from build123d import *

# Parameters (mm, degrees)
IZIM1_W                      = 50.7
IZIM1_H                      = 48.2
Y_KSEKLIK_EKSTR_ZYON1_DEPTH  = 26.7
IZIM2_R                      = 8.7
Y_KSEKLIK_EKSTR_ZYON2_DEPTH  = 0.5
Y_KSEKLIK_EKSTR_ZYON3_DEPTH  = 11.9
IZIM4_R                      = 16.5
Y_KSEKLIK_EKSTR_ZYON4_DEPTH  = 0.9
IZIM5_R                      = 18
Y_KSEKLIK_EKSTR_ZYON5_DEPTH  = 0.9
Y_KSEKLIK_EKSTR_ZYON6_DEPTH  = 36
Y_KSEKLIK_EKSTR_ZYON7_DEPTH  = 17
Y_KSEKLIK_EKSTR_ZYON8_START  = 17
Y_KSEKLIK_EKSTR_ZYON8_DEPTH  = 17
IZIM9_W                      = 14.75
IZIM9_H                      = 70
KES_EKSTR_ZYON1_DEPTH        = 30.160746911
IZIM10_W                     = 14.75
IZIM10_H                     = 70
KES_EKSTR_ZYON2_DEPTH        = 30.160746911
IZIM11_W                     = 50.7
IZIM11_H                     = 48.2
Y_KSEKLIK_EKSTR_ZYON9_DEPTH  = 9.3
Y_KSEKLIK_EKSTR_ZYON10_START = 20
Y_KSEKLIK_EKSTR_ZYON10_DEPTH = 20
IZIM13_W                     = 9.75
IZIM13_H                     = 10.2
Y_KSEKLIK_EKSTR_ZYON11_DEPTH = 26.5
Y_KSEKLIK_EKSTR_ZYON12_DEPTH = 42.2
Y_KSEKLIK_EKSTR_ZYON13_START = -42.2
Y_KSEKLIK_EKSTR_ZYON13_DEPTH = 42.2
IZIM16_W                     = 29
IZIM16_H                     = 34.79
Y_KSEKLIK_EKSTR_ZYON14_DEPTH = 9.9
Y_KSEKLIK_EKSTR_ZYON15_DEPTH = 8.5
Y_KSEKLIK_EKSTR_ZYON16_DEPTH = 8.5
IZIM19_W                     = 6.3
IZIM19_H                     = 0.8
Y_KSEKLIK_EKSTR_ZYON17_DEPTH = 12
DRAFT1_ANGLE                 = 50
IZIM20_W                     = 5
IZIM20_H                     = 7.5
IZIM21_W                     = 5
IZIM21_H                     = 7.5
IZIM22_W                     = 5
IZIM22_H                     = 7.5
IZIM23_W                     = 5
IZIM23_H                     = 7.5
IZIM24_W                     = 5.2
IZIM24_H                     = 2.6
M20_BO_LUKLU_DELIK1_D        = 24
M20_BO_LUKLU_DELIK1_DEPTH    = 33.25
M27_BO_LUKLU_DELIK2_D        = 30.291
M27_BO_LUKLU_DELIK2_DEPTH    = 33.249
FEDER1_START                 = -30
FEDER1_DEPTH                 = 9.75
PAH1_SIZE                    = 1.479
RADYUS1_R                    = 0.8
RADYUS2_R                    = 2
RADYUS3_R                    = 5
RADYUS4_R                    = 5.1
RADYUS5_R                    = 7
RADYUS6_R                    = 8.16
L_EK1_SCALE                  = 0.31


# Read off the part's stored shape, not the designer's step: Feder1
with BuildPart() as part:
    # Çizim1 → Yükseklik-Ekstrüzyon1 (new body)
    with BuildSketch(Plane(origin=(18, 0, 0), x_dir=(0, 0, -1), z_dir=(1, 0, 0))):
        with Locations((-0.35, 68.8)):
            Rectangle(IZIM1_W, IZIM1_H)
    extrude(amount=-Y_KSEKLIK_EKSTR_ZYON1_DEPTH)

    # Çizim2 → Yükseklik-Ekstrüzyon2 (add)
    with BuildSketch(Plane.XZ.offset(-44.7)):
        with Locations(Location((0, 0, 0), (0, 0, 180))):
            Circle(IZIM2_R)
    extrude(amount=Y_KSEKLIK_EKSTR_ZYON2_DEPTH)

    # Çizim3 → Yükseklik-Ekstrüzyon3 (add)
    with BuildSketch(Plane(origin=(0, 44.2, 0), x_dir=(1, 0, 0), z_dir=(0, 1, 0))):
        Polygon((-18, 10.392304845), (-18, -10.392304845), (0, -20.784609691), (18, -10.392304845), (18, 10.392304845), (0, 20.784609691), align=None)
    extrude(amount=-Y_KSEKLIK_EKSTR_ZYON3_DEPTH)

    # Çizim4 → Yükseklik-Ekstrüzyon4 (add)
    with BuildSketch(Plane.XZ.offset(-32.3)):
        with Locations(Location((0, 0, 0), (0, 0, 270))):
            Circle(IZIM4_R)
    extrude(amount=Y_KSEKLIK_EKSTR_ZYON4_DEPTH)

    # Çizim5 → Yükseklik-Ekstrüzyon5 (add)
    with BuildSketch(Plane(origin=(0, 31.4, 0), x_dir=(1, 0, 0), z_dir=(0, 1, 0))):
        with Locations(Location((0, 0, 0), (0, 0, 90))):
            Circle(IZIM5_R)
    extrude(amount=-Y_KSEKLIK_EKSTR_ZYON5_DEPTH)

    # Çizim6 → Yükseklik-Ekstrüzyon6 (add)
    with BuildSketch(Plane.XY.offset(18)):
        with BuildLine():
            Line((-13.564659966, -21), (13.564659966, -21))
            ThreePointArc((13.564659966, -21), (17.201870235, -18.14099392), (20.25, -14.660746911))
            Line((20.25, -14.660746911), (35, -14.660746911))
            Line((35, -14.660746911), (35, 30.5))
            Line((35, 30.5), (0, 30.5))
            Line((0, 30.5), (-35, 30.5))
            Line((-35, 30.5), (-35, -14.660746911))
            Line((-35, -14.660746911), (-20.25, -14.660746911))
            ThreePointArc((-20.25, -14.660746911), (-17.201870235, -18.14099392), (-13.564659966, -21))
        make_face()
    extrude(amount=-Y_KSEKLIK_EKSTR_ZYON6_DEPTH)

    # Çizim7 → Yükseklik-Ekstrüzyon7 (add)
    with BuildSketch(Plane(origin=(0, 0, -18), x_dir=(-1, 0, 0), z_dir=(0, 0, -1))):
        with BuildLine():
            Line((13.564659966, -21), (-13.564659966, -21))
            ThreePointArc((-13.564659966, -21), (-17.201870235, -18.14099392), (-20.25, -14.660746911))
            Line((-20.25, -14.660746911), (-35, -14.660746911))
            Line((-35, -14.660746911), (-35, 30.5))
            Line((-35, 30.5), (35, 30.5))
            Line((35, 30.5), (35, -14.660746911))
            Line((35, -14.660746911), (20.25, -14.660746911))
            ThreePointArc((20.25, -14.660746911), (17.201870235, -18.14099392), (13.564659966, -21))
        make_face()
    extrude(amount=Y_KSEKLIK_EKSTR_ZYON7_DEPTH)

    # Çizim8 → Yükseklik-Ekstrüzyon8 (add)
    with BuildSketch(Plane.XY.offset(18).offset(Y_KSEKLIK_EKSTR_ZYON8_START)):
        with BuildLine():
            Line((13.564659966, -21), (-13.564659966, -21))
            ThreePointArc((-13.564659966, -21), (-17.201870235, -18.14099392), (-20.25, -14.660746911))
            Line((-20.25, -14.660746911), (-35, -14.660746911))
            Line((-35, -14.660746911), (-35, 30.5))
            Line((-35, 30.5), (35, 30.5))
            Line((35, 30.5), (35, -14.660746911))
            Line((35, -14.660746911), (20.25, -14.660746911))
            ThreePointArc((20.25, -14.660746911), (17.201870235, -18.14099392), (13.564659966, -21))
        make_face()
    extrude(amount=-Y_KSEKLIK_EKSTR_ZYON8_DEPTH)

    # Çizim9 → Kes-Ekstrüzyon1 (cut)
    with BuildSketch(Plane.XZ.offset(14.660746911)):
        with Locations((27.625, 0)):
            Rectangle(IZIM9_W, IZIM9_H)
    extrude(amount=-KES_EKSTR_ZYON1_DEPTH, mode=Mode.SUBTRACT)

    # Çizim10 → Kes-Ekstrüzyon2 (cut)
    with BuildSketch(Plane.XZ.offset(14.660746911)):
        with Locations((-27.625, 0)):
            Rectangle(IZIM10_W, IZIM10_H)
    extrude(amount=-KES_EKSTR_ZYON2_DEPTH, mode=Mode.SUBTRACT)

    # Çizim11 → Yükseklik-Ekstrüzyon9 (add)
    with BuildSketch(Plane.ZY.offset(8.7)):
        with Locations((0.35, 68.8)):
            Rectangle(IZIM11_W, IZIM11_H)
    extrude(amount=Y_KSEKLIK_EKSTR_ZYON9_DEPTH)

    # Çizim12 → Yükseklik-Ekstrüzyon10 (add)
    with BuildSketch(Plane.XY.offset(35).offset(Y_KSEKLIK_EKSTR_ZYON10_START)):
        with BuildLine():
            Line((-20.25, -14.660746911), (-20.25, 17.715834237))
            ThreePointArc((-20.25, 17.715834237), (0, 22), (20.25, 17.715834237))
            Line((20.25, 17.715834237), (20.25, -14.660746911))
            ThreePointArc((20.25, -14.660746911), (17.201870235, -18.14099392), (13.564659966, -21))
            Line((13.564659966, -21), (-13.564659966, -21))
            ThreePointArc((-13.564659966, -21), (-17.201870235, -18.14099392), (-20.25, -14.660746911))
        make_face()
    extrude(amount=-Y_KSEKLIK_EKSTR_ZYON10_DEPTH)

    # Çizim13 → Yükseklik-Ekstrüzyon11 (add)
    with BuildSketch(Plane.XZ.offset(-15.5)):
        with Locations((25.125, 15.1)):
            Rectangle(IZIM13_W, IZIM13_H)
    extrude(amount=Y_KSEKLIK_EKSTR_ZYON11_DEPTH)

    # Çizim14 → Yükseklik-Ekstrüzyon12 (add)
    with BuildSketch(Plane(origin=(0, 89.9, 0), x_dir=(1, 0, 0), z_dir=(0, 1, 0))):
        with BuildLine():
            Line((-18, -8.717797887), (-18, 8.717797887))
            ThreePointArc((-18, 8.717797887), (-20, 0), (-18, -8.717797887))
        make_face()
    extrude(amount=-Y_KSEKLIK_EKSTR_ZYON12_DEPTH)

    # Çizim15 → Yükseklik-Ekstrüzyon13 (add)
    with BuildSketch(Plane.XZ.offset(-47.7).offset(Y_KSEKLIK_EKSTR_ZYON13_START)):
        with BuildLine():
            Line((18, 8.717797887), (18, -8.717797887))
            ThreePointArc((18, -8.717797887), (20, 0), (18, 8.717797887))
        make_face()
    extrude(amount=Y_KSEKLIK_EKSTR_ZYON13_DEPTH)

    # Çizim16 → Yükseklik-Ekstrüzyon14 (add)
    with BuildSketch(Plane.XY.offset(25.7)):
        with Locations((0, 75.495)):
            Rectangle(IZIM16_W, IZIM16_H)
    extrude(amount=Y_KSEKLIK_EKSTR_ZYON14_DEPTH)

    # Çizim17 → Yükseklik-Ekstrüzyon15 (add)
    with BuildSketch(Plane.XY.offset(35.6)):
        Polygon((-9.4, 81.4), (-7.6, 81.4), (-7.6, 80.6), (-8.6, 80.6), (-8.6, 77.4), (-7.6, 77.4), (-7.6, 76.6), (-9.4, 76.6), align=None)
    extrude(amount=Y_KSEKLIK_EKSTR_ZYON15_DEPTH)

    # Çizim18 → Yükseklik-Ekstrüzyon16 (add)
    with BuildSketch(Plane.XY.offset(35.6)):
        Polygon((7.6, 77.4), (8.6, 77.4), (8.6, 80.6), (7.6, 80.6), (7.6, 81.4), (9.4, 81.4), (9.4, 76.6), (7.6, 76.6), align=None)
    extrude(amount=Y_KSEKLIK_EKSTR_ZYON16_DEPTH)

    # Çizim19 → Yükseklik-Ekstrüzyon17 (add)
    with BuildSketch(Plane.XY.offset(35.6)):
        with Locations((0, 70)):
            Rectangle(IZIM19_W, IZIM19_H)
    extrude(amount=Y_KSEKLIK_EKSTR_ZYON17_DEPTH)

    # Draft1
    draft1_faces = [part.faces().sort_by_distance(p)[0] for p in [
        (25.125, 2.25, 10),
    ]]
    draft(draft1_faces, Plane(origin=(0, -11, 0), x_dir=(0, 0, -1), z_dir=(0, -1, 0)), DRAFT1_ANGLE)

    # Çizim20 → Döndür1 (revolve)
    with BuildSketch(Plane.XY.offset(26.25), mode=Mode.PRIVATE) as d_nd_r1_sk:
        with Locations((-23.75, 34.25)):
            Rectangle(IZIM20_W, IZIM20_H)
    revolve(d_nd_r1_sk.sketch.rotate(Axis((-26.25, 38, 26.25), (0, -1, 0)), 270), axis=Axis((-26.25, 38, 26.25), (0, -1, 0)))

    # Çizim21 → Döndür2 (revolve)
    with BuildSketch(Plane.XY.offset(-26.25), mode=Mode.PRIVATE) as d_nd_r2_sk:
        with Locations((-23.75, 34.25)):
            Rectangle(IZIM21_W, IZIM21_H)
    revolve(d_nd_r2_sk.sketch.rotate(Axis((-26.25, 38, -26.25), (0, -1, 0)), 270), axis=Axis((-26.25, 38, -26.25), (0, -1, 0)))

    # Çizim22 → Döndür3 (revolve)
    with BuildSketch(Plane.XY.offset(-26.25), mode=Mode.PRIVATE) as d_nd_r3_sk:
        with Locations((28.75, 34.25)):
            Rectangle(IZIM22_W, IZIM22_H)
    revolve(d_nd_r3_sk.sketch.rotate(Axis((26.25, 38, -26.25), (0, -1, 0)), 270), axis=Axis((26.25, 38, -26.25), (0, -1, 0)))

    # Çizim23 → Döndür4 (revolve)
    with BuildSketch(Plane.XY.offset(26.25), mode=Mode.PRIVATE) as d_nd_r4_sk:
        with Locations((28.75, 34.25)):
            Rectangle(IZIM23_W, IZIM23_H)
    revolve(d_nd_r4_sk.sketch.rotate(Axis((26.25, 38, 26.25), (0, -1, 0)), 270), axis=Axis((26.25, 38, 26.25), (0, -1, 0)))

    # Çizim24 → Döndür5 (revolve)
    with BuildSketch(Plane(origin=(0, 0, 0), x_dir=(-1, 0, 0), z_dir=(0, 0, -1)), mode=Mode.PRIVATE) as d_nd_r5_sk:
        with Locations((-2.6, 94.2)):
            Rectangle(IZIM24_W, IZIM24_H)
    revolve(d_nd_r5_sk.sketch.rotate(Axis((0, 92.9, 0), (0, 1, 0)), 90), axis=Axis((0, 92.9, 0), (0, 1, 0)))

    # M20 Boşluklu Delik1
    with Locations(Plane.XY.offset(55)):
        with Locations((0, 0)):
            Hole(M20_BO_LUKLU_DELIK1_D / 2, depth=M20_BO_LUKLU_DELIK1_DEPTH)

    # M27 Boşluklu Delik2
    with Locations(Plane(origin=(0, 0, -35), x_dir=(-1, 0, 0), z_dir=(0, 0, -1))):
        with Locations((0, 0)):
            Hole(M27_BO_LUKLU_DELIK2_D / 2, depth=M27_BO_LUKLU_DELIK2_DEPTH)

    # Feder1 outline → Feder1 (add)
    with BuildSketch(Plane.YZ.offset(FEDER1_START)):
        Polygon((15.5, 19.826070485), (-9.313312955, 19.826070485), (-12.686687045, 12.591846402), (15.5, -20.999739147), align=None)
    extrude(amount=FEDER1_DEPTH)

    # Pah1
    pah1_edges = [part.edges().sort_by_distance(p)[0] for p in [
        (12, 0, 55),
        (-15.1455, 0, -35),
    ]]
    chamfer(pah1_edges, length=PAH1_SIZE)

    # Radyus1
    radyus1_edges = [part.edges().sort_by_distance(p)[0] for p in [
        (-9.4, 81.4, 39.85),
        (-9.4, 76.6, 39.85),
        (9.4, 76.6, 39.85),
        (9.4, 81.4, 39.85),
    ]]
    fillet(radyus1_edges, radius=RADYUS1_R)

    # Radyus2
    radyus2_edges = [part.edges().sort_by_distance(p)[0] for p in [
        (-18, 68.8, -25),
        (-18, 68.8, 25.7),
        (-14.5, 92.89, 30.65),
        (-14.5, 58.1, 30.65),
        (14.5, 58.1, 30.65),
        (14.5, 92.89, 30.65),
        (18, 68.8, 25.7),
        (18, 68.8, -25),
    ]]
    fillet(radyus2_edges, radius=RADYUS2_R)

    # Radyus3
    radyus3_edges = [part.edges().sort_by_distance(p)[0] for p in [
        (-18, 38.25, -10.392304845),
        (0, 38.25, -20.784609691),
        (18, 38.25, -10.392304845),
        (18, 38.25, 10.392304845),
        (0, 38.25, 20.784609691),
        (-18, 38.25, 10.392304845),
    ]]
    fillet(radyus3_edges, radius=RADYUS3_R)

    # Radyus4
    radyus4_edges = [part.edges().sort_by_distance(p)[0] for p in [
        (25.125, -11, 20.2),
    ]]
    fillet(radyus4_edges, radius=RADYUS4_R)

    # Radyus5
    radyus5_edges = [part.edges().sort_by_distance(p)[0] for p in [
        (35, 23, 35),
        (-35, 23, -35),
        (35, 23, -35),
        (-35, 23, 35),
    ]]
    fillet(radyus5_edges, radius=RADYUS5_R)

    # Radyus6
    radyus6_edges = [part.edges().sort_by_distance(p)[0] for p in [
        (25.125, -11, 10),
    ]]
    fillet(radyus6_edges, radius=RADYUS6_R)


with BuildPart() as part_1:
    # Ölçek1: scaled about (0.014012089, 30.59302606, 5.902020233)
    add(part.part.scale(L_EK1_SCALE).moved(Location((0.009668341, 21.109187981, 4.072393961))))


solid = part_1.part
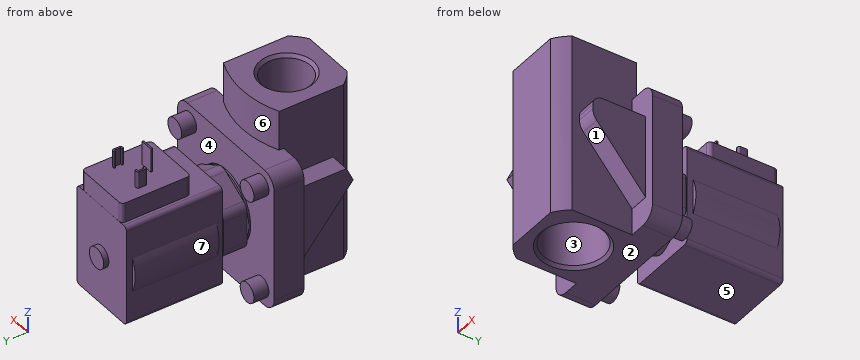
CAD build for the part. Positions are in the model's coordinates, mm. Face numbers are marked on the shaded views. A direction names the side the tool comes from. Round coordinates to 2 decimals unless told otherwise and drop trailing zeros. Write each loop counter-clockwise with the first axis right and the second up, starting at its lowest first coordinate (ties: lowest second). Pieces come first, ordered by that corner, then holes. Notation, with made-up numbers: M -26.5,58.5 L 2.5,58.5 A18 cw 2.5,86.5 Z; hole C 69.25,-28 d2. An arc over 180 degrees is marked long. Use a Markdown table: item, result. Add a question column.
1. Pull direction Y, two halves, no side cores. Call the marked faces 1, 2 and 3: released by +Y, released by -Y, zero draft, split by the parting line, or undercut.
2. Drill centre lines: probe 1 along Y at (x, z) = (2.75, 12); probe 2 along Y at (x, z) = (-4, 9.75); probe 3 along Z at (x, y) = (4.75, 43.5). Where is each one in solid material? Low to high.
3. Slice it at D-D on y = 47. Give the cut face in (x, z).
4. Flat gauge pins, fed straight in: P1, Ø4, axis at y = 44.5, z = 14.5, coming from the -X side; P2, Ø4, axis at y = 20.5, z = 3.5, coming from the +X side; P3, Ø1.6, axis at x = 0, z = 17, coming from the +Y side. Where does each tip first touch, or does it go through?
5. Slice it at C-C on y = 38. Give the cut face in (x, z), then the cut area to 3 significant figures.
6. 3-axis set-ups, long thin cutter, end or side, ignore diameter. For the marked faces 4, 5, 6 and 7: which of +Z, -Z, +X, -X, +Y, -Y reach the whole face in a straight line?
7. Slice it at A-A on z = -0.5. Give the number of separate pieces and of enclosed holes in the cut face, then the cut area to 3 significant figures.
Reply:
| question | item | result |
|---|---|---|
| 1 | face 1 | released by -Y |
| 1 | face 2 | zero draft |
| 1 | face 3 | undercut |
| 2 | probe 1 | y = 14.6 to 18.59, 23.62 to 30.56, 34.97 to 49.91 |
| 2 | probe 2 | y = 14.6 to 30.56, 34.97 to 49.91 |
| 2 | probe 3 | z = -3.68 to 12.04 |
| 3 | outline | M -5.57,-3.06 A0.62 ccw -4.95,-3.68 L 4.97,-3.68 A0.62 ccw 5.59,-3.06 L 5.59,1.37 A6.2 ccw 5.59,6.77 L 5.59,11.42 A0.62 ccw 4.97,12.04 L 4.5,12.04 L 4.5,15.11 L -4.49,15.11 L -4.49,12.04 L -4.95,12.04 A0.62 ccw -5.57,11.42 L -5.57,6.77 A6.2 ccw -5.57,1.37 Z |
| 4 | P1 | stops at x = -4.49 |
| 4 | P2 | stops at x = 9.31 |
| 4 | P3 | stops at y = 42.93 |
| 5 | outline | M -5.57,-3.06 A0.62 ccw -4.95,-3.68 L 4.97,-3.68 A0.62 ccw 5.59,-3.06 L 5.59,1.37 A6.2 ccw 5.59,6.77 L 5.59,11.42 A0.62 ccw 4.97,12.04 L -4.95,12.04 A0.62 ccw -5.57,11.42 L -5.57,6.77 A6.2 ccw -5.57,1.37 Z |
| 5 | area | 180 mm^2 |
| 6 | face 4 | none |
| 6 | face 5 | -Z, +X, -X, +Y |
| 6 | face 6 | +Z |
| 6 | face 7 | -X, +Y |
| 7 | separate pieces | 2 |
| 7 | enclosed holes | 1 |
| 7 | area | 374 mm^2 |
